from build123d import *

# Parameters (mm, degrees)
SKETCH2_W           = 60
SKETCH2_H           = 70
SKETCH2_R           = 4.5
BOSS_EXTRUDE1_DEPTH = 4
SKETCH3_W           = 60
SKETCH3_H           = 25
BOSS_EXTRUDE2_DEPTH = 12
FILLET1_R           = 2
SKETCH4_R           = 2.5
CUT_EXTRUDE1_DEPTH  = 28


with BuildPart() as part:
    # Sketch2 → Boss-Extrude1 (new body)
    with BuildSketch(Plane.XY):
        with Locations((-11.05214497, -10.673076923)):
            Rectangle(SKETCH2_W, SKETCH2_H)
        with Locations((-11.05214497, 1.316923077)):
            Circle(SKETCH2_R, mode=Mode.SUBTRACT)
    extrude(amount=BOSS_EXTRUDE1_DEPTH)

    # Sketch3 → Boss-Extrude2 (add)
    with BuildSketch(Plane(origin=(0, 0, 0), x_dir=(-1, 0, 0), z_dir=(0, 0, -1))):
        with Locations((11.05214497, -33.173076923)):
            Rectangle(SKETCH3_W, SKETCH3_H)
    extrude(amount=BOSS_EXTRUDE2_DEPTH)

    # Fillet1
    fillet1_edges = [part.edges().sort_by_distance(p)[0] for p in [
        (-41.05214497, -20.673076923, -6),
        (18.94785503, -20.673076923, -6),
        (-11.05214497, -20.673076923, -12),
    ]]
    fillet(fillet1_edges, radius=FILLET1_R)

    # Sketch4 → Cut-Extrude1 (cut)
    with BuildSketch(Plane(origin=(0, -20.673076923, 0), x_dir=(1, 0, 0), z_dir=(0, 1, 0))):
        with Locations(Location((-29.05214497, 5, 0), (0, 0, 270))):
            Circle(SKETCH4_R)
        with Locations(Location((6.94785503, 5, 0), (0, 0, 270))):
            Circle(SKETCH4_R)
    extrude(amount=-CUT_EXTRUDE1_DEPTH, mode=Mode.SUBTRACT)


solid = part.part
Could you check a few things on this model? Use its own coordinates, in mm. A direction names the side the tool comes from. Coordinates: 2 decimals unless noted, no trailing zeros. Order: outer loops, then holes, each group sorted by start corner. A loop starts at its lowest first (then second) coordinate and runs counter-clockwise, first axis right, second up. Notation, with made-up numbers: (-0.75, 30.5) -> (21.25, 30.5) arc R12 ccw to (21.25, 35.5) -> close; hole circle Ø9 at (49, -33.5). An arc over 180 degrees is marked (long way). One line per question, with ' | ' between items.
Q1. On a 3-axis mill with a long thin cutter (end or side, diameter ignored), from which of +Z, -Z, +X, -X, +Y, -Y can I reach the whole of each face in a straight line? I mean faces 1 (the face through (-11, -20.673, -5)), 2 (the face through (-40.48, -21.27, -6.08)), 3 (the face through (-11, -10, 4)). Say none if no direction works.
Return value:
face 1: -Z, +X, -X, +Y | face 2: -Z, -X, +Y | face 3: +Z, +X, -X, +Y, -Y
Q2. Imagine slicing it at C-C on z = -1. Please give me the cut outline in (x, y).
Return value:
outline: (-41.05, -45.67) -> (18.95, -45.67) -> (18.95, -22.67) arc R2 ccw to (16.95, -20.67) -> (-39.05, -20.67) arc R2 ccw to (-41.05, -22.67) -> close
Q3. Imagine slicing it at D-D on y = -30.5. Please give me the cut outline in (x, z).
Return value:
outline: (-41.05, -12) -> (18.95, -12) -> (18.95, 4) -> (-41.05, 4) -> close; hole circle Ø5 at (-29.05, -5); hole circle Ø5 at (6.95, -5)
Q4. Imagine slicing it at B-B on x = -9. Please give me the cut outline in (y, z), and give its area (3 significant figures).
Return value:
outline: (-45.67, -12) -> (-22.67, -12) arc R2 ccw to (-20.67, -10) -> (-20.67, 0) -> (-2.69, 0) -> (-2.69, 4) -> (-45.67, 4) -> close; (5.32, 0) -> (24.33, 0) -> (24.33, 4) -> (5.32, 4) -> close | area: 547 mm²
Q5. I'm going to push flat-ended pins straight in: P1, Ø1.5, axis at x = -22, y = 14.5, coming from the -Z side; P2, Ø2, axis at x = -9.5, z = -8, coming from the +Y side; P3, Ø8, axis at x = -1.5, z = -2, coming from the +Y side. Where does each tip first touch, or does it pass through?
Return value:
P1: z = 0 | P2: y = -20.67 | P3: y = 24.33
Q6. Thinking about a two-plate mould opening in Y: for faces 4 (the face through (18.4, -21.3, -6.1)), 5 (the face through (18.948, -27, -2)), 6 (the face through (-15.55, 1.51, 1.97)), which applies, pulls with the +Y half, pulls with the -Y half, needs draft (parallel to the pull), parting line crosses it, or undercut?
Return value:
face 4: pulls with the +Y half | face 5: needs draft | face 6: undercut
Q7. If I drill on L1, parallel to X at y = -40.5, z = -5; L2, parallel to Z at x = 16, y = 18.5; L3, parallel to Y at x = -35.5, z = -9, over which ranges is the centre line in solid material (lowest first)?
Return value:
L1: -41.05 to -31.55, -26.55 to 4.45, 9.45 to 18.95 | L2: 0 to 4 | L3: -45.67 to -20.67
Q8. Imagine slicing it at A-A on z = -5. Please give me the cut outline in (x, y).
Return value:
outline: (-41.05, -45.67) -> (-31.55, -45.67) -> (-31.55, -20.67) -> (-39.05, -20.67) arc R2 ccw to (-41.05, -22.67) -> close; (-26.55, -45.67) -> (4.45, -45.67) -> (4.45, -20.67) -> (-26.55, -20.67) -> close; (9.45, -45.67) -> (18.95, -45.67) -> (18.95, -22.67) arc R2 ccw to (16.95, -20.67) -> (9.45, -20.67) -> close
